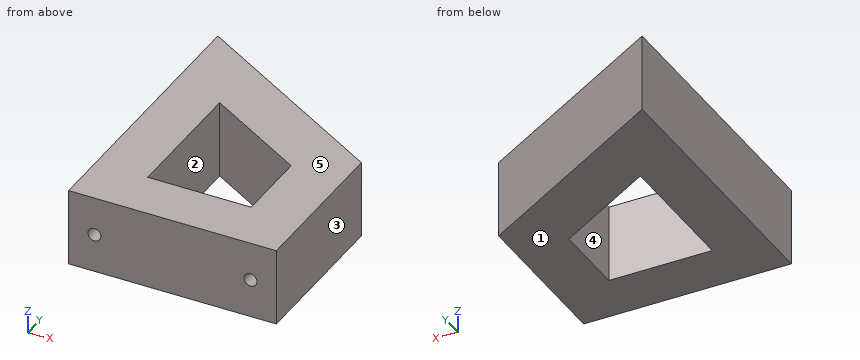
```python
from build123d import *

# Parameters (mm, degrees)
F1_DEPTH = 19
F2_R     = 1.0795
F3_DEPTH = 19.05
F5_D     = 3.175
F5_DEPTH = 16.51
F5_TIP   = 0.9538662327


with BuildPart() as f1:
    # F0 (on Top) → F1 (new body)
    with BuildSketch(Plane.XY):
        Polygon((0, 69.3), (0, 0), (51, 0), (51, 39.5), align=None)
        Polygon((38.1, 12.7), (12.7, 12.7), (12.7, 46.1200160448), (38.1, 31.2784474173), align=None, mode=Mode.SUBTRACT)
    extrude(amount=F1_DEPTH)

    # F2 (on face) → F3 (join)
    with BuildSketch(Plane.XZ):
        with Locations((6.35, 9.5)):
            Circle(F2_R)
        with Locations((44.65, 9.5)):
            Circle(F2_R)
    extrude(amount=-F3_DEPTH)

    # F5
    with Locations(Plane.XZ):
        with Locations((6.35, 9.5), (44.65, 9.5)):
            Hole(F5_D / 2, depth=F5_DEPTH)
            with Locations((0, 0, -(F5_DEPTH + F5_TIP / 2))):  # 118° drill point
                Cone(0, F5_D / 2, F5_TIP, mode=Mode.SUBTRACT)


solid = f1.part
```
Design review of the part built by this model. Coordinates are the model's own, in mm. Face numbers are marked on the shaded views. A direction names the side the tool comes from. Give positions to 0.01 mm unless a question says otherwise; leave off trailing zeros. Order: outer loops, then holes, each group sorted by start corner. A loop starts at its lowest first (then second) coordinate and runs counter-clockwise, first axis right, second up. Notation, with made-up numbers: (-39.5, 31) -> (0.5, 31) arc R20 cw to (0.5, 66) -> close; hole circle Ø4 at (-20, -10). An arc over 180 degrees is marked (long way). Write item = value, one per line. Start each with the question number.
(1) We need section B-B on x = 22. Write out the cut boundary in (y, z), plus the area to 3 significant figures.
(2) We need section D-D on y = 11. State how many separate pieces and enclosed holes the cut face has, plus the area to 3 significant figures.
(3) We need section C-C on z = 6.75. Write out the cut boundary in (x, y), plus the area to 3 significant figures.
(4) To check wall thickness, follow line 1 along X through (y, z) = (9.75, 9.5); line 2 along Z through (x, y) = (44.65, 5); line 3 along X through (y, z) = (28.5, 16). State the ranges of each line that lie inside material, in increasing order.
(5) We need section A-A on y = 28.5. Write out the cut boundary in (x, z).
(6) For pin 1 (6 mm diameter, centred on x = 22.5, z = 10, fed in from +Y); pin 2 (9.5 mm diameter, centred on x = 21.5, z = 14, fed in from +Y); pin 3 (2 mm diameter, centred on x = 22.5, z = 13.5, fed in from +Y), all flat-tipped, find the tip position at first contact; note any pin that passes through.
(7) For the marked faces 1 and 2, list the 3-axis set-ups (+Z, -Z, +X, -X, +Y, -Y) from which the entire face can be reached by the end or side of a thin tool; tool diameter is ignored.
(8) Mouldability with a two-part tool opening along X and no side actions: class the marked faces 3, 4 and 5 as +X half, -X half, draft (parallel to the pull), parting line (faces both ways), or undercut.
Numbers:
q1.outline = (0, 0) -> (12.7, 0) -> (12.7, 19) -> (0, 19) -> close; (40.69, 0) -> (56.45, 0) -> (56.45, 19) -> (40.69, 19) -> close
q1.area = 541 mm^2
q2.separate_pieces = 1
q2.enclosed_holes = 2
q2.area = 953 mm^2
q3.outline = (0, 0) -> (51, 0) -> (51, 39.5) -> (0, 69.3) -> close; hole (12.7, 12.7) -> (38.1, 12.7) -> (38.1, 31.28) -> (12.7, 46.12) -> close
q3.area = 2,110 mm^2
q4.line_1 = 0 to 4.76, 7.94 to 43.06, 46.24 to 51
q4.line_2 = 0 to 7.91, 11.09 to 19
q4.line_3 = 0 to 12.7, 38.1 to 51
q5.outline = (0, 0) -> (12.7, 0) -> (12.7, 19) -> (0, 19) -> close; (38.1, 0) -> (51, 0) -> (51, 19) -> (38.1, 19) -> close
q6.pin_1 = 57.91
q6.pin_2 = 59.51
q6.pin_3 = 56.74
q7.face_1 = -Z, +X, -X, +Y, -Y
q7.face_2 = +Z, -Z
q8.face_3 = +X half
q8.face_4 = undercut
q8.face_5 = draft
